Verification items for this drawing (mm, ordinates from the low corner). A direction names the side the tool comes from. Give positions to 0.01 mm unless a question says otherwise; leave off trailing zeros. Loops run counter-clockwise (first coordinate to the right, second up) from the corner with the lowest first, then second, coordinate; pieces in that order, holes last. Notation, with made-up numbers: M 18.25,37.25 L 63.25,37.25 A6 ccw 63.25,48.25 Z; hole C 41,74 d1. An arc over 180 degrees is marked long. Put each result on its own line as item: value. Start each with the question number.
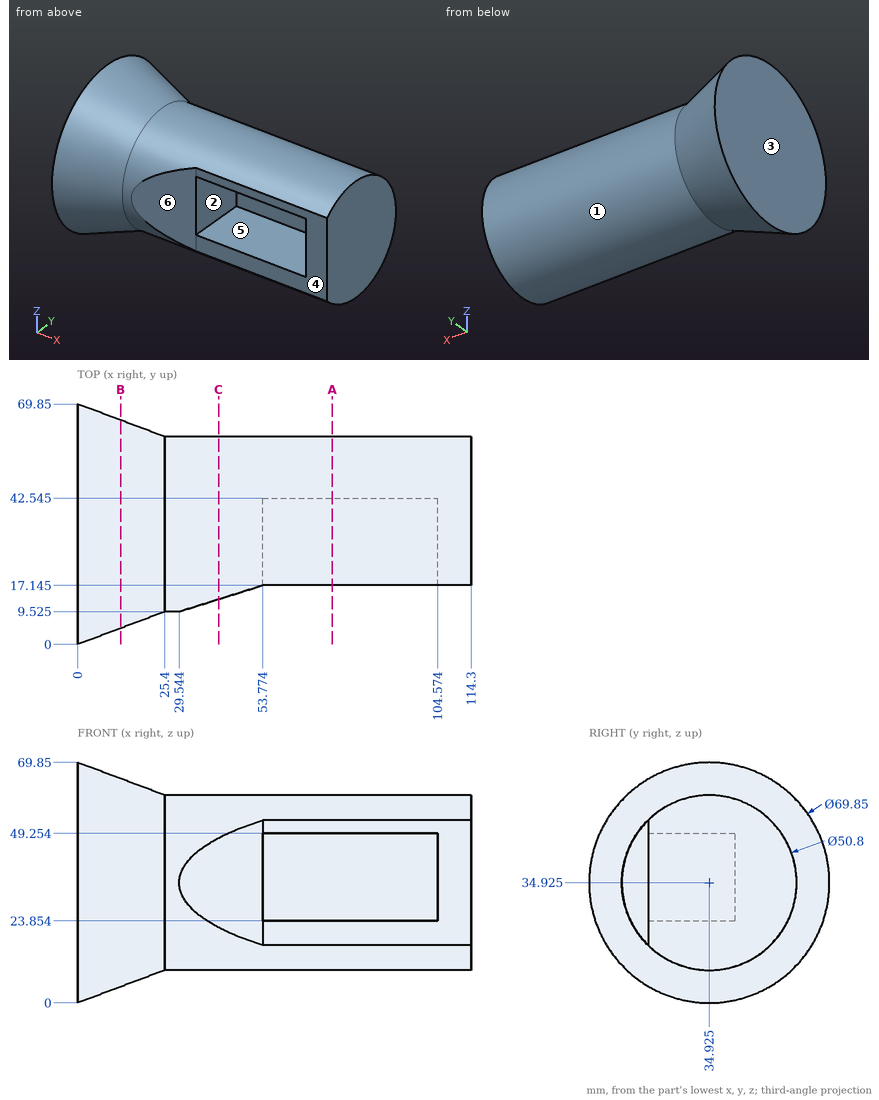
Q1. Set-up check for the marked faces 1, 2 and 3: record each of +Z, -Z, +X, -X, +Y, -Y from which the full face is reachable in a straight line by a thin tool's end or side.
Q2. Cross-section at A-A, the plane x = 74. Record the boundary of the cut face in (y, z) (1 decimal), then the cut area to 3 significant figures.
Q3. Scan lines: L1, parallel to X at y = 38, z = 38.5; L2, parallel to Z at x = 91.5, y = 27; L3, parallel to Z at x = 96, y = 33.5 (1 decimal). Record each from-to range of solid material in increasing order.
Q4. Go/stop test with flat-tipped pins: pin 1 (12 mm diameter, centred on x = 37, y = 32.5, fed in from -Z) (3 decimals); pin 2 (10 mm diameter, centred on x = 61, y = 61.5, fed in from +Z); pin 3 (12 mm diameter, centred on x = 37.5, y = 25.5, fed in from +Z). Record where each tip stops, or that it passes through.
Q5. Cross-section at B-B, the plane x = 12.5. Record the boundary of the cut face in (y, z) (1 decimal).
Q6. Cross-section at C-C, the plane x = 41. Record the boundary of the cut face in (y, z) (1 decimal).
Q7. Release check for a two-part mould opening along X. For the marked faces 4, 5 and 6 record: pulls with the +X half, pulls with the -X half, needs draft (parallel to the pull), parting line crosses it, or undercut.
Ans:
1. face 1: +X
1. face 2: -Y
1. face 3: +Z, -Z, -X, +Y, -Y
2. outline: M 17.1,16.8 A25.4 ccw long 17.1,53.1 L 17.1,49.3 L 42.5,49.3 L 42.5,23.9 L 17.1,23.9 Z
2. area: 1,190 mm^2
3. L1: x = 0 to 53.77, 104.57 to 114.3
3. L2: z = 10.79 to 23.85, 49.25 to 59.06
3. L3: z = 9.6 to 23.9, 49.3 to 60.3
4. pin 1: stops at z = 9.525
4. pin 2: stops at z = 48.33
4. pin 3: stops at z = 60.09
5. outline: C 34.9,34.9 d60.5
6. outline: M 13.1,21.9 A25.4 ccw long 13.1,48 Z
7. face 4: needs draft
7. face 5: undercut
7. face 6: pulls with the +X half
